Verification items for the finished model (mm, model axes). A direction names the side the tool comes from. Give positions to 0.01 mm unless a question says otherwise; leave off trailing zeros. Write each loop counter-clockwise with the first axis right and the second up, starting at its lowest first coordinate (ties: lowest second). Pieces come first, ordered by that corner, then holes.
from build123d import *

# Parameters (mm, degrees)
BOSS_EXTRUDE1_DEPTH                             = 4
SKETCH3_W                                       = 29.5
SKETCH3_H                                       = 19.5
SKETCH3_W_2                                     = 27
CUT_EXTRUDE3_DEPTH                              = 195.527632999
BOSS_EXTRUDE2_DEPTH                             = 4
FILLET5_R                                       = 5
CSK_FOR_M3_FLAT_HEAD_MACHINE_SCREW1_D           = 3.3
CSK_FOR_M3_FLAT_HEAD_MACHINE_SCREW1_CSINK_D     = 6
CSK_FOR_M3_FLAT_HEAD_MACHINE_SCREW1_CSINK_ANGLE = 90
SKETCH8_R                                       = 1.65
CUT_EXTRUDE4_DEPTH                              = 204.958218206
FILLET6_R                                       = 5


with BuildPart() as part:
    # Sketch1 → Boss-Extrude1 (new body)
    with BuildSketch(Plane.XY):
        with BuildLine():
            Line((0, 0), (135, 0))
            Line((135, 0), (135, 140))
            Line((135, 140), (0, 140))
            Line((0, 140), (0, 97.072711728))
            ThreePointArc((0, 97.072711728), (-0.211219914, 95.028259617), (-0.835956887, 93.070173307))
            Line((-0.835956887, 93.070173307), (-9.164043113, 74.002538421))
            ThreePointArc((-9.164043113, 74.002538421), (-10, 70), (-9.164043113, 65.997461579))
            Line((-9.164043113, 65.997461579), (-0.835956887, 46.929826693))
            ThreePointArc((-0.835956887, 46.929826693), (-0.211219914, 44.971740383), (0, 42.927288272))
            Line((0, 42.927288272), (0, 0))
        make_face()
    extrude(amount=BOSS_EXTRUDE1_DEPTH)

    # Sketch3 → Cut-Extrude3 (cut, through all)
    with BuildSketch(Plane.XY.offset(4)):
        with Locations((14.75, 9.75)):
            Rectangle(SKETCH3_W, SKETCH3_H)
        with Locations((70, 9.75)):
            Rectangle(SKETCH3_W_2, SKETCH3_H)
        with Locations((125.25, 130.25)):
            Rectangle(SKETCH3_W, SKETCH3_H)
        with Locations((125.25, 9.75)):
            Rectangle(SKETCH3_W, SKETCH3_H)
        with Locations((14.75, 130.25)):
            Rectangle(SKETCH3_W, SKETCH3_H)
        with Locations((70, 130.25)):
            Rectangle(SKETCH3_W_2, SKETCH3_H)
    extrude(amount=-CUT_EXTRUDE3_DEPTH, mode=Mode.SUBTRACT)

    # Sketch9 → Boss-Extrude2 (add)
    with BuildSketch(Plane(origin=(0, 0, 0), x_dir=(-1, 0, 0), z_dir=(0, 0, -1))):
        Polygon((-140, 98.5), (-148.266499161, 98.5), (-148.266499161, 86.5), (-135, 83.5), (-135, 105.5), (-135, 120.5), (-140, 120.5), align=None)
        Polygon((-140, 19.5), (-140, 41.5), (-148.266499161, 41.5), (-148.266499161, 53.5), (-135, 56.5), (-135, 34.5), (-135, 19.5), align=None)
    extrude(amount=-BOSS_EXTRUDE2_DEPTH)

    # Fillet5
    fillet5_edges = [part.edges().sort_by_distance(p)[0] for p in [
        (135, 83.5, 2),
        (148.266499161, 86.5, 2),
        (148.266499161, 98.5, 2),
        (148.266499161, 41.5, 2),
        (148.266499161, 53.5, 2),
        (135, 56.5, 2),
    ]]
    fillet(fillet5_edges, radius=FILLET5_R)

    # CSK for M3 Flat Head Machine Screw1 (through all)
    with Locations(Plane(origin=(0, 0, 0), x_dir=(-1, 0, 0), z_dir=(0, 0, -1))):
        with Locations((-10, 70), (-130, 92), (-130, 48)):
            CounterSinkHole(CSK_FOR_M3_FLAT_HEAD_MACHINE_SCREW1_D / 2, CSK_FOR_M3_FLAT_HEAD_MACHINE_SCREW1_CSINK_D / 2, counter_sink_angle=CSK_FOR_M3_FLAT_HEAD_MACHINE_SCREW1_CSINK_ANGLE)

    # Sketch8 → Cut-Extrude4 (cut, through all)
    with BuildSketch(Plane(origin=(0, 0, 0), x_dir=(-1, 0, 0), z_dir=(0, 0, -1))):
        with Locations((3, 70)):
            Circle(SKETCH8_R)
        with Locations((-143, 92)):
            Circle(SKETCH8_R)
        with Locations((-143, 48)):
            Circle(SKETCH8_R)
    extrude(amount=-CUT_EXTRUDE4_DEPTH, mode=Mode.SUBTRACT)

    # Fillet6
    fillet6_edges = [part.edges().sort_by_distance(p)[0] for p in [
        (83.5, 120.5, 2),
        (56.5, 120.5, 2),
        (140, 120.5, 2),
        (140, 19.5, 2),
        (0, 19.5, 2),
        (29.5, 19.5, 2),
        (56.5, 19.5, 2),
        (83.5, 19.5, 2),
        (110.5, 19.5, 2),
        (110.5, 120.5, 2),
        (29.5, 120.5, 2),
        (0, 120.5, 2),
    ]]
    fillet(fillet6_edges, radius=FILLET6_R)


solid = part.part
Item 1: Sectioned sample at B-B on x = 76. Record the cut outline in (y, z), then the cut area to 3 significant figures.
Answer key:
outline: (19.5, 0) - (120.5, 0) - (120.5, 4) - (19.5, 4) - close
area: 404 mm2
Item 2: Scan lines: line 1 along Y through (x, z) = (130, 2.65); line 2 along X through (y, z) = (47, 1.85); line 3 along Y through (x, z) = (10, 2.85). Record each from-to range of solid material in increasing order.
Answer key:
line 1: y = 19.5 to 46.35, 49.65 to 90.35, 93.65 to 120.5
line 2: x = -0.87 to 128.69, 131.31 to 141.69, 144.31 to 148.27
line 3: y = 19.5 to 68.35, 71.65 to 120.5
Item 3: Release check for a two-part mould opening along Y. For faces 5 (the face through (29.5, 7, 2)), 6 (the face through (141.67, 54.99, 1.97)), 7 (the face through (82.07, 122, 1.97)) record: released by +Y, released by -Y, zero draft, split by the parting line, or undercut.
Answer key:
face 5: zero draft
face 6: undercut
face 7: released by +Y
Item 4: Sectioned sample at A-A on y = 21.5. Record the cut outline in (x, z), then the cut area to 3 significant figures.
Answer key:
outline: (1, 0) - (139, 0) - (139, 4) - (1, 4) - close
area: 552 mm2
Item 5: Sectioned sample at C-C on z = 3.1. State how many separate pieces and enclosed holes the cut face has, then the cut area to 3 significant figures.
Answer key:
separate pieces: 1
enclosed holes: 6
area: 16,500 mm2
Item 6: Set-up check for faces 1 (the face through (15, 120.5, 2)), 2 (the face through (142, 98.5, 2)), 3 (the face through (82.07, 18, 1.97)), 4 (the face through (140, 33, 2)): record each of +Z, -Z, +X, -X, +Y, -Y from which the full face is reachable in a straight line by a thin tool's end or side.
Answer key:
face 1: +Z, -Z, -X, +Y
face 2: +Z, -Z, +X, +Y
face 3: +Z, -Z, -Y
face 4: +Z, -Z, +X, -Y
Item 7: Depth check by flat-ended pin: pin 1 (2 mm diameter, centred on y = 5.5, z = 1, fed in from -X); pin 2 (10 mm diameter, centred on x = 121, y = 111.5, fed in from -Z); pin 3 (1.5 mm diameter, centred on y = 105, z = 3, fed in from -X); pin 4 (2 mm diameter, centred on y = 4, z = 1.5, fed in from +X). Enter the tip coordinate at first touch or a pass-through.
Answer key:
pin 1: stops at x = 29.5
pin 2: stops at z = 0
pin 3: stops at x = 0
pin 4: stops at x = 110.5
